Could you check a few things on this model? Use its own coordinates, in mm. A direction names the side the tool comes from. Coordinates: 2 decimals unless noted, no trailing zeros. Loops run counter-clockwise (first coordinate to the right, second up) from the corner with the lowest first, then second, coordinate; pieces in that order, holes last.
1) If I drill on line 1 along X through (y, z) = (57, 2.2); line 2 along Y through (x, z) = (5, 2.05); line 3 along Y through (x, z) = (139, 2.85), over which ranges is the centre line in solid material (lowest first)?
2) Imagine slicing it at B-B on x = 61.5. Please give me the cut outline in (y, z).
3) Imagine slicing it at D-D on x = 146.5. Please give me the cut outline in (y, z), plus the area to 3 significant figures.
4) Will these pins go through, and if not, where does the flat tip stop? P1, Ø1.5, axis at x = 99.5, z = 1.5, coming from the -Y side; P2, Ø4, axis at x = 93.5, y = 12, coming from the -Z side; P3, Ø0.9, axis at y = 41, z = 1.5, coming from the +X side; P4, Ø0.9, axis at y = 47, z = 2, coming from the -X side.
5) Imagine slicing it at C-C on z = 0.9. Give the number of separate pieces and of enclosed holes in the cut face, plus the area to 3 significant figures.
6) Thinking about a two-plate mould opening in Y: for faces 1 (the face through (-3, 36, 1)), 2 (the face through (45, 58, 2)), 3 (the face through (127, -3, 1)), which applies, released by +Y, released by -Y, zero draft, split by the parting line, or undercut?
7) For faces 4 (the face through (58, 0, 1)), 5 (the face through (117, 45.108, 1)), 6 (the face through (-1, 20.554, 1)), 7 (the face through (57.9, 23.4, 1.5)), 8 (the face through (138, -2, 1)), which set-ups out of +Z, -Z, +X, -X, +Y, -Y let a thin tool reach every point of the face, with its end or its side?
8) Imagine slicing it at A-A on x = 21. Please give me the cut outline in (y, z).
```python
from build123d import *

# Parameters (mm, degrees)
SKETCH1_W           = 115.6
SKETCH1_H           = 72
BOSS_EXTRUDE1_DEPTH = 3
CUT_EXTRUDE1_REACH  = 5
SKETCH2_W           = 42
SKETCH2_H           = 22
SKETCH3_W           = 3
SKETCH3_H           = 10.29
SKETCH3_H_2         = 8.964
BOSS_EXTRUDE2_DEPTH = 3
SKETCH6_W           = 45.782864491
SKETCH6_H           = 27.18
BOSS_EXTRUDE4_DEPTH = 3
SKETCH8_W           = 23
SKETCH8_H           = 3
BOSS_EXTRUDE5_DEPTH = 3


with BuildPart() as part:
    # Sketch1 → Boss-Extrude1 (new body)
    with BuildSketch(Plane.XY):
        with Locations((57.8, 36)):
            Rectangle(SKETCH1_W, SKETCH1_H)
        Polygon((16.514285714, 38.123846184), (15.508587017, 35.297440316), (32.022872733, 29.421286499), (33.02857143, 32.247692367), align=None, mode=Mode.SUBTRACT)
        Polygon((49.542857146, 26.37153855), (48.537158448, 23.545132682), (65.051444164, 17.668978865), (66.057142861, 20.495384733), align=None, mode=Mode.SUBTRACT)
        Polygon((82.571428577, 14.619230916), (81.56572988, 11.792825048), (98.080015595, 5.916671232), (99.085714292, 8.743077099), align=None, mode=Mode.SUBTRACT)
    extrude(amount=BOSS_EXTRUDE1_DEPTH)

    # Sketch2 → Cut-Extrude1 (cut, up to next)
    with BuildSketch(Plane.XY.offset(3), mode=Mode.PRIVATE) as cut_extrude1_sk1:
        with Locations((24, 58)):
            Rectangle(SKETCH2_W, SKETCH2_H)
    cut_extrude1_tool1 = extrude(cut_extrude1_sk1.sketch, amount=-CUT_EXTRUDE1_REACH, mode=Mode.PRIVATE) & part.part
    add(cut_extrude1_tool1.solids().sort_by_distance((24, 58, 3))[0], mode=Mode.SUBTRACT)

    # Sketch3 → Boss-Extrude2 (add)
    with BuildSketch(Plane(origin=(0, 0, 0), x_dir=(-1, 0, 0), z_dir=(0, 0, -1))):
        with Locations((1.5, 56.569285714)):
            Rectangle(SKETCH3_W, SKETCH3_H)
        with Locations((1.5, 35.989285714)):
            Rectangle(SKETCH3_W, SKETCH3_H)
        with Locations((1.5, 15.409285714)):
            Rectangle(SKETCH3_W, SKETCH3_H)
        with Locations((-117.1, 58.554)):
            Rectangle(SKETCH3_W, SKETCH3_H_2)
        with Locations((-117.1, 40.626)):
            Rectangle(SKETCH3_W, SKETCH3_H_2)
    extrude(amount=-BOSS_EXTRUDE2_DEPTH)

    # Sketch6 → Boss-Extrude4 (add)
    with BuildSketch(Plane(origin=(0, 0, 0), x_dir=(-1, 0, 0), z_dir=(0, 0, -1))):
        with Locations((-138.491432246, 13.59)):
            Rectangle(SKETCH6_W, SKETCH6_H)
    extrude(amount=-BOSS_EXTRUDE4_DEPTH)

    # Sketch8 → Boss-Extrude5 (add)
    with BuildSketch(Plane(origin=(0, 0, 0), x_dir=(-1, 0, 0), z_dir=(0, 0, -1))):
        with Locations((-34.5, -1.5)):
            Rectangle(SKETCH8_W, SKETCH8_H)
        with Locations((-80.5, -1.5)):
            Rectangle(SKETCH8_W, SKETCH8_H)
        with Locations((-126.5, -1.5)):
            Rectangle(SKETCH8_W, SKETCH8_H)
    extrude(amount=-BOSS_EXTRUDE5_DEPTH)


solid = part.part
```
Filled in:
1. line 1: x = -3 to 3, 45 to 118.6
1. line 2: y = 0 to 47, 69 to 72
1. line 3: y = 0 to 27.18
2. outline: (0, 0) - (18.93, 0) - (18.93, 3) - (0, 3) - close; (22.12, 0) - (72, 0) - (72, 3) - (22.12, 3) - close
3. outline: (0, 0) - (27.18, 0) - (27.18, 3) - (0, 3) - close
3. area: 81.5 mm2
4. P1: stops at y = 0
4. P2: stops at z = 0
4. P3: stops at x = 118.6
4. P4: stops at x = 0
5. separate pieces: 1
5. enclosed holes: 4
5. area: 8,840 mm2
6. face 1: zero draft
6. face 2: undercut
6. face 3: released by -Y
7. face 4: +Z, -Z, -Y
7. face 5: +Z, -Z, +X
7. face 6: +Z, -Z, -X
7. face 7: +Z, -Z
7. face 8: +Z, -Z, +X, -Y
8. outline: (0, 0) - (33.34, 0) - (33.34, 3) - (0, 3) - close; (36.53, 0) - (47, 0) - (47, 3) - (36.53, 3) - close; (69, 0) - (72, 0) - (72, 3) - (69, 3) - close
